Could you check a few things on this model? Use its own coordinates, in mm. Face numbers are marked on the shaded views. A direction names the side the tool comes from. Round coordinates to 2 decimals unless told otherwise and drop trailing zeros. Order: outer loops, then holes, each group sorted by start corner. A loop starts at its lowest first (then second) coordinate and runs counter-clockwise, first axis right, second up. Notation, with made-up numbers: (29, -17.75) - (68, -17.75) arc R12 cw to (68, -1.75) - close; hole circle Ø5 at (4, -24.75). An arc over 180 degrees is marked (long way). Use one line per item in the form item = value.
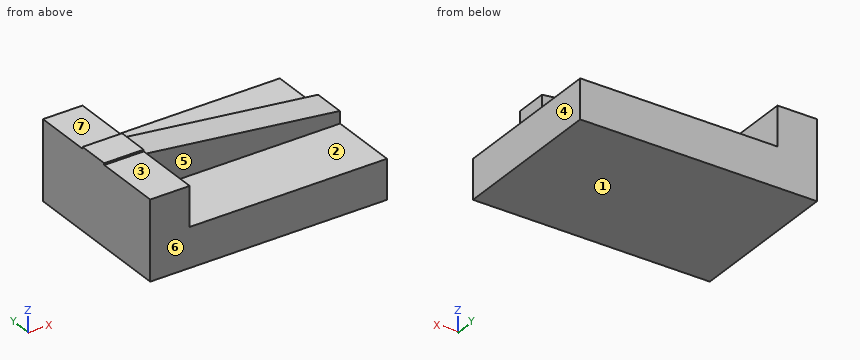
from build123d import *

# Parameters (mm, degrees)
F1_DEPTH = 101.6
F2_W     = 20.5739997327
F2_H     = 25.399999693
F3_DEPTH = 151.638
F4_DEPTH = 2.286
F6_DEPTH = 32.512
F7_DEPTH = 2.794


with BuildPart() as f1:
    # F0 (on Front) → F1 (new body)
    with BuildSketch(Plane.XZ):
        Polygon((0, 50.8), (0, 0), (152.4, 0), (152.4, 25.4), (25.4, 25.4), (25.4, 50.8), align=None)
    extrude(amount=F1_DEPTH)

    # F2 (on Right) → F3 (join)
    with BuildSketch(Plane.YZ):
        with Locations((-47.7519985288, 38.735001348)):
            Rectangle(F2_W, F2_H)
    extrude(amount=F3_DEPTH)

    # F4 (cut): a face of the model
    f4_faces = [f1.faces().sort_by_distance(p)[0] for p in [
        (75.819, -47.7519985288, 51.4350011945),
    ]]
    extrude(f4_faces, amount=-F4_DEPTH, mode=Mode.SUBTRACT)

    # F5 (on face) → F6 (cut)
    with BuildSketch(Plane.XZ.offset(58.0389983952)):
        Polygon((151.638, 49.1490011945), (25.4, 49.1490011945), (151.638, 33.8758528233), align=None)
    extrude(amount=-F6_DEPTH, mode=Mode.SUBTRACT)

    # F7 (add): a face of the model
    f7_faces = [f1.faces().sort_by_distance(p)[0] for p in [
        (12.7, -47.7519985288, 49.1490011945),
    ]]
    extrude(f7_faces, amount=F7_DEPTH)


solid = f1.part
Item 1: Imagine slicing it at C-C on x = 63.5. Please give me the cut outline in (y, z) (3 decimals), plus the area to 3 significant figures.
Found:
outline = (-101.6, 0) - (0, 0) - (0, 25.4) - (-101.6, 25.4) - close; (-58.039, 26.035) - (-37.465, 26.035) - (-37.465, 44.539) - (-58.039, 44.539) - close
area = 2,960 mm2
Item 2: Imagine slicing it at A-A on x = 22.5. Please give me the cut outline in (y, z) (3 decimals).
Found:
outline = (-101.6, 0) - (0, 0) - (0, 50.8) - (-37.465, 50.8) - (-37.465, 51.943) - (-58.039, 51.943) - (-58.039, 50.8) - (-101.6, 50.8) - close
Item 3: If we mould it in two halves opening along Z, with no side actions, what happens to the marked faces 1, 2, 3 and 4? For each: released by +Z, released by -Z, zero draft, split by the parting line, or undercut.
Found:
face_1 = released by -Z
face_2 = undercut
face_3 = released by +Z
face_4 = zero draft
Item 4: Imagine slicing it at D-D on z = 47. Please give me the cut outline in (x, y) (3 decimals), plus the area to 3 significant figures.
Found:
outline = (0, -101.6) - (25.4, -101.6) - (25.4, -58.039) - (43.162, -58.039) - (43.162, -37.465) - (25.4, -37.465) - (25.4, 0) - (0, 0) - close
area = 2,950 mm2
Item 5: Will these pins go through, and if not, where does the flat tip stop? P1, Ø8, axis at x = 128.5, y = -10.5, coming from the +Z side; P2, Ø21, axis at y = -75, z = 37, coming from the +X side; P3, Ø2.5, axis at y = -49.5, z = 29.5, coming from the +X side; P4, Ø2, axis at x = 110, y = -24, coming from the -Z side.
Found:
P1 = 25.4
P2 = 25.4
P3 = 151.64
P4 = 0
Item 6: For the marked faces 5, 6 and 7, which set-ups out of +Z, -Z, +X, -X, +Y, -Y let a thin tool reach every point of the face, with its end or its side?
Found:
face_5 = +Z, +X, -Y
face_6 = +Z, -Z, +X, -X, -Y
face_7 = +Z, +X, -X, +Y
Item 7: I need wall thicknesses on L1, parallel to X at y = -22, z = 50; L2, parallel to Y at x = 116.5, z = 28.5 (3 decimals); L3, parallel to Z at x = 13.5, y = -33. Which ranges of each line are inside material? Lowest first, please.
Found:
L1 = 0 to 25.4
L2 = -58.039 to -37.465
L3 = 0 to 50.8
Item 8: Imagine slicing it at B-B on y = -48. Please give me the cut outline in (x, z) (3 decimals).
Found:
outline = (0, 0) - (152.4, 0) - (152.4, 25.4) - (25.4, 25.4) - (25.4, 26.035) - (151.638, 26.035) - (151.638, 33.876) - (25.4, 49.149) - (25.4, 51.943) - (0, 51.943) - close
